Design review of the part built by this model. Coordinates are the model's own, in mm. Give positions to 0.01 mm unless a question says otherwise; leave off trailing zeros. Loops run counter-clockwise (first coordinate to the right, second up) from the corner with the lowest first, then second, coordinate; pieces in that order, holes last. Notation, with made-up numbers: M 39,-12 L 93,-12 A3 cw 93,-7 Z; hole C 69,9 d3. An arc over 180 degrees is marked long. Use one line per item in the form item = value. Start each with the question number.
from build123d import *

# Parameters (mm, degrees)
SKETCH1_R           = 150
BOSS_EXTRUDE1_DEPTH = 2.5


with BuildPart() as part:
    # Sketch1 → Boss-Extrude1 (new body, symmetric)
    with BuildSketch(Plane(origin=(0, 0, 0), x_dir=(1, 0, 0), z_dir=(0, 1, 0))):
        Circle(SKETCH1_R)
        with BuildLine():
            Line((2.525, -129.975476052), (2.525, -140))
            Line((2.525, -140), (-2.975, -140))
            Line((-2.975, -140), (-2.975, -129.965954677))
            ThreePointArc((-2.975, -129.965954677), (-92.082878446, -91.764609176), (-129.975476052, -2.525))
            Line((-129.975476052, -2.525), (-140, -2.525))
            Line((-140, -2.525), (-140, 2.975))
            Line((-140, 2.975), (-129.965954677, 2.975))
            ThreePointArc((-129.965954677, 2.975), (-91.764609176, 92.082878446), (-2.525, 129.975476052))
            Line((-2.525, 129.975476052), (-2.525, 140))
            Line((-2.525, 140), (2.975, 140))
            Line((2.975, 140), (2.975, 129.965954677))
            ThreePointArc((2.975, 129.965954677), (92.082878446, 91.764609176), (129.975476052, 2.525))
            Line((129.975476052, 2.525), (140, 2.525))
            Line((140, 2.525), (140, -2.975))
            Line((140, -2.975), (129.965954677, -2.975))
            ThreePointArc((129.965954677, -2.975), (91.764609176, -92.082878446), (2.525, -129.975476052))
        make_face(mode=Mode.SUBTRACT)
    extrude(amount=BOSS_EXTRUDE1_DEPTH, both=True)


solid = part.part
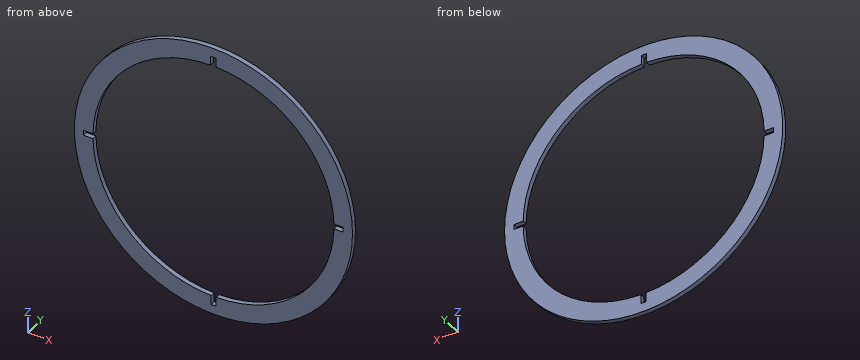
Q1. Take a section at A-A on y = -1.6. Give the boundary of the cut face in (x, z) (3 decimals).
Q2. Clearance check with flat-ended pins moving along their axes: pin 1 Ø2.5 at (x, y) = (-137, 0) entering from +Z; pin 2 Ø2.5 at (x, y) = (135, 0) entering from +Z; pin 3 Ø2.5 at (y, z) = (0, -1) entering from -X; pin 4 Ø1 at (y, z) = (-2, 63) entering from +X. State where each tip first meets the part, or that it passes through.
Q3. Wall thickness on probe 1 along X at (y, z) = (0.05, -86); probe 2 along X at (y, z) = (1.8, -33); probe 3 along Z at (x, y) = (91, -0.05): over which ranges is each line inside the solid? List them lowest first.
Q4. Take a section at B-B on z = -113.5. Give the boundary of the cut face in (x, y), plus the area to 3 significant figures.
Q5. Take a section at C-C on x = -53.5. Give the boundary of the cut face in (y, z), plus the area to 3 significant figures.
Response values:
q1.outline = C 0,0 d300; hole M -140,-2.975 L -129.966,-2.975 A130 ccw -2.525,-129.975 L -2.525,-140 L 2.975,-140 L 2.975,-129.966 A130 ccw 129.975,-2.525 L 140,-2.525 L 140,2.975 L 129.966,2.975 A130 ccw 2.525,129.975 L 2.525,140 L -2.975,140 L -2.975,129.966 A130 ccw -129.975,2.525 L -140,2.525 Z
q2.pin_1 = 63.81
q2.pin_2 = 67.9
q2.pin_3 = -150
q2.pin_4 = 136.36
q3.probe_1 = -122.9 to -97.49, 97.49 to 122.9
q3.probe_2 = -146.32 to -125.74, 125.74 to 146.32
q3.probe_3 = -119.24 to -92.84, 92.84 to 119.24
q4.outline = M -98.07,-2.5 L -63.39,-2.5 L -63.39,2.5 L -98.07,2.5 Z; M 63.39,-2.5 L 98.07,-2.5 L 98.07,2.5 L 63.39,2.5 Z
q4.area = 347 mm^2
q5.outline = M -2.5,-140.13 L 2.5,-140.13 L 2.5,-118.48 L -2.5,-118.48 Z; M -2.5,118.48 L 2.5,118.48 L 2.5,140.13 L -2.5,140.13 Z
q5.area = 217 mm^2
